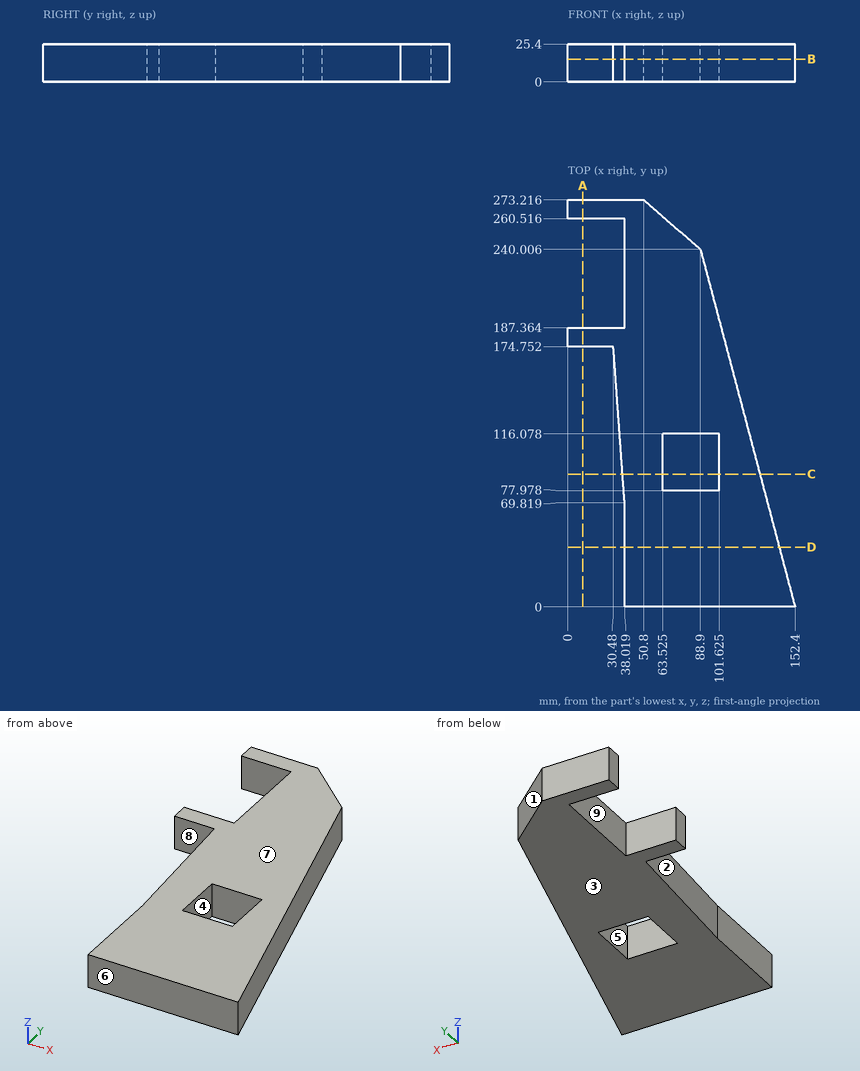
Verification items for this drawing (mm, ordinates from the low corner). A direction names the side the tool comes from. Round coordinates to 2 decimals unless told otherwise and drop trailing zeros. Loops run counter-clockwise (first coordinate to the right, second up) from the corner with the lowest first, then second, coordinate; pieces in that order, holes last. Notation, with made-up numbers: (0, 4.25) -> (45, 4.25) arc R8 ccw to (45, 10.25) -> close; hole circle Ø6 at (-5.75, 33.5). An arc over 180 degrees is marked (long way). Answer in a Markdown table with one row per item.
Q1. Sectioned sample at A-A on x = 10. Enter the section's corners in (y, z).
Data:
| item | result |
|---|---|
| outline | (174.75, 0) -> (187.36, 0) -> (187.36, 25.4) -> (174.75, 25.4) -> close; (260.52, 0) -> (273.22, 0) -> (273.22, 25.4) -> (260.52, 25.4) -> close |
Q2. Sectioned sample at C-C on y = 89. Enter the section's corners in (x, z) (1 decimal), then the cut area to 3 significant figures.
Data:
| item | result |
|---|---|
| outline | (36.6, 0) -> (63.5, 0) -> (63.5, 25.4) -> (36.6, 25.4) -> close; (101.6, 0) -> (128.9, 0) -> (128.9, 25.4) -> (101.6, 25.4) -> close |
| area | 1,370 mm^2 |
Q3. Release check for a two-part mould opening along Y. For the marked faces 1, 2, 3 and 4 record: released by +Y, released by -Y, zero draft, split by the parting line, or undercut.
Data:
| item | result |
|---|---|
| face 1 | released by +Y |
| face 2 | released by -Y |
| face 3 | zero draft |
| face 4 | undercut |
Q4. Go/stop test with flat-tipped pins: P1, Ø7.5, axis at y = 221.5, z = 18.5, coming from the -X side; P2, Ø7.5, axis at y = 96, z = 16, coming from the -X side; P3, Ø10, axis at y = 119.5, z = 15.5, coming from the +X side. Record where each tip stops, or that it passes through.
Data:
| item | result |
|---|---|
| P1 | stops at x = 38.02 |
| P2 | stops at x = 35.87 |
| P3 | stops at x = 122.11 |
Q5. Thickness scan on L1, parallel to Y at x = 26, z = 14.75; L2, parallel to X at y = 240, z = 18.25; L3, parallel to Y at x = 85.5, z = 24.25. Record the ranges inside material, lowest first.
Data:
| item | result |
|---|---|
| L1 | y = 174.75 to 187.36, 260.52 to 273.22 |
| L2 | x = 38.02 to 88.9 |
| L3 | y = 0 to 77.98, 116.08 to 242.97 |
Q6. Set-up check for the marked faces 5, 6, 7, 8 and 9: record each of +Z, -Z, +X, -X, +Y, -Y from which the full face is reachable in a straight line by a thin tool's end or side.
Data:
| item | result |
|---|---|
| face 5 | +Z, -Z |
| face 6 | +Z, -Z, +X, -X, -Y |
| face 7 | +Z, +X, -X, +Y, -Y |
| face 8 | +Z, -Z, -X, -Y |
| face 9 | +Z, -Z, -X |
Q7. Sectioned sample at B-B on z = 15.25. Enter the section's corners in (x, y) (1 decimal), then the cut area to 3 significant figures.
Data:
| item | result |
|---|---|
| outline | (0, 174.8) -> (30.5, 174.8) -> (38, 69.8) -> (38, 0) -> (152.4, 0) -> (88.9, 240) -> (50.8, 273.2) -> (0, 273.2) -> (0, 260.5) -> (38, 260.5) -> (38, 187.4) -> (0, 187.4) -> close; hole (63.5, 78) -> (101.6, 78) -> (101.6, 116.1) -> (63.5, 116.1) -> close |
| area | 20,800 mm^2 |
Q8. Sectioned sample at D-D on y = 40. Enter the section's corners in (x, z).
Data:
| item | result |
|---|---|
| outline | (38.02, 0) -> (141.82, 0) -> (141.82, 25.4) -> (38.02, 25.4) -> close |
